Answer from the drawing. Dimensions are ordinates in mm from the lowest x, y and z of the part. A direction names the side the tool comes from. Round coordinates to 2 decimals unless told otherwise and drop trailing zeros. Write each loop counter-clockwise with the first axis right and the second up, starting at its lowest first coordinate (ties: lowest second). Pieces come first, ordered by that corner, then holes. Notation, with made-up numbers: (30.5, 51.5) - (52.5, 51.5) arc R28 ccw to (52.5, 71.5) - close; hole circle Ø9 at (-34.5, 29.5). An arc over 180 degrees is marked (long way). Write item = value, one per line. Start each with the question number.
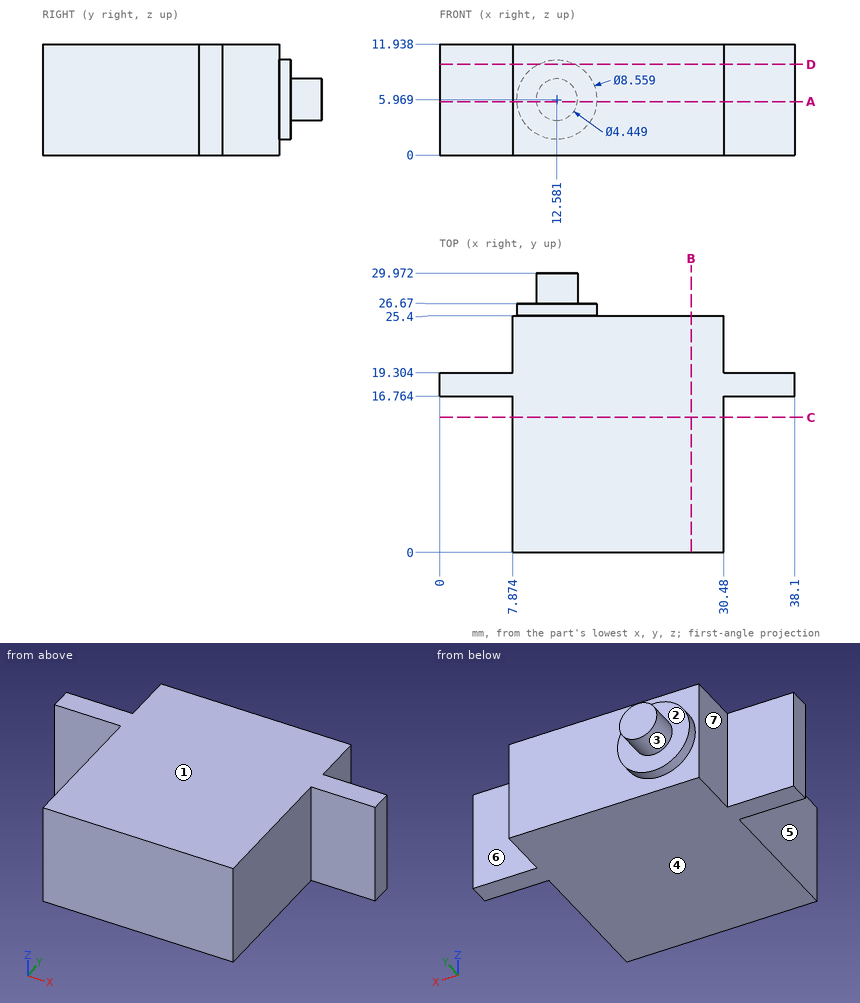
1. Find section B-B on x = 27. Give the vertices of the cut face in (y, z).
2. For a pull along Z with two mould halves and no side action, classify the marked faces 1, 2, 3 and 4 as released by +Z, released by -Z, zero draft, split by the parting line, or undercut.
3. Consider line 1 (X direction, y = 15.5, z = 1.25); line 2 (Y direction, x = 15, z = 4); line 3 (Y direction, x = 16.5, z = 4). Determine where each line is inside the solid, lowest interval first.
4. Each of these flat-tipped pins is pushed along its axis until it touches: pin 1 (4 mm diameter, centred on x = 3, z = 9, fed in from -Y); pin 2 (6.5 mm diameter, centred on y = 24, z = 8.5, fed in from -X); pin 3 (6.5 mm diameter, centred on y = 23.5, z = 7.5, fed in from +X). Where does it stop, or does it pass through?
5. Find section D-D on z = 9.75. Give the vertices of the cut face in (x, y), plus the area to 3 significant figures.
6. Which of the six approach directions +Z, -Z, +X, -X, +Y, -Y give full straight-line access (tool end or side, diameter ignored) to the marked faces 5, 6 and 7?
7. Find section C-C on y = 14.5. Give the vertices of the cut face in (x, z).
8. Find section A-A on z = 5.75. Give the vertices of the cut face in (x, y) (1 decimal).
Answer key:
q1.outline = (0, 0) - (25.4, 0) - (25.4, 11.94) - (0, 11.94) - close
q2.face_1 = released by +Z
q2.face_2 = zero draft
q2.face_3 = split by the parting line
q2.face_4 = released by -Z
q3.line_1 = 7.87 to 30.48
q3.line_2 = 0 to 26.67
q3.line_3 = 0 to 25.4
q4.pin_1 = 16.76
q4.pin_2 = 7.87
q4.pin_3 = 30.48
q5.outline = (0, 16.76) - (7.87, 16.76) - (7.87, 0) - (30.48, 0) - (30.48, 16.76) - (38.1, 16.76) - (38.1, 19.3) - (30.48, 19.3) - (30.48, 25.4) - (14.59, 25.4) - (14.59, 26.67) - (10.58, 26.67) - (10.58, 25.4) - (7.87, 25.4) - (7.87, 19.3) - (0, 19.3) - close
q5.area = 619 mm²
q6.face_5 = +Z, -Z, -X, -Y
q6.face_6 = +Z, -Z, +X, +Y
q6.face_7 = +Z, -Z, -X, +Y
q7.outline = (7.87, 0) - (30.48, 0) - (30.48, 11.94) - (7.87, 11.94) - close
q8.outline = (0, 16.8) - (7.9, 16.8) - (7.9, 0) - (30.5, 0) - (30.5, 16.8) - (38.1, 16.8) - (38.1, 19.3) - (30.5, 19.3) - (30.5, 25.4) - (16.9, 25.4) - (16.9, 26.7) - (14.8, 26.7) - (14.8, 30) - (10.4, 30) - (10.4, 26.7) - (8.3, 26.7) - (8.3, 25.4) - (7.9, 25.4) - (7.9, 19.3) - (0, 19.3) - close
